from build123d import *

# Parameters (mm, degrees)
SKETCH1_R           = 2.66
BOSS_EXTRUDE1_DEPTH = 3
CUT_EXTRUDE1_DEPTH  = 2
SKETCH3_R           = 1.5
BOSS_EXTRUDE2_DEPTH = 10


with BuildPart() as part:
    # Sketch1 → Boss-Extrude1 (new body)
    with BuildSketch(Plane(origin=(0, 0, 0), x_dir=(1, 0, 0), z_dir=(0, 1, 0))):
        with Locations(Location((0, 0, 0), (0, 0, 270))):
            Circle(SKETCH1_R)
    extrude(amount=BOSS_EXTRUDE1_DEPTH)

    # Sketch2 → Cut-Extrude1 (cut)
    with BuildSketch(Plane(origin=(0, 3, 0), x_dir=(1, 0, 0), z_dir=(0, 1, 0))):
        Polygon((1.732050808, 0), (0.866025404, 1.5), (-0.866025404, 1.5), (-1.732050808, 0), (-0.866025404, -1.5), (0.866025404, -1.5), align=None)
    extrude(amount=-CUT_EXTRUDE1_DEPTH, mode=Mode.SUBTRACT)

    # Sketch3 → Boss-Extrude2 (add)
    with BuildSketch(Plane.XZ):
        with Locations(Location((0, 0, 0), (0, 0, 90))):
            Circle(SKETCH3_R)
    extrude(amount=BOSS_EXTRUDE2_DEPTH)


solid = part.part
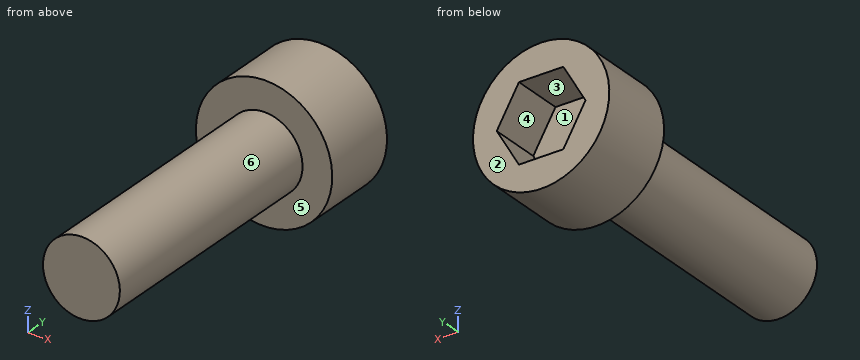
The listing builds one solid part. Answer for the finished solid, in the listing's coordinates (mm). Face numbers are marked on the shaded views. A direction names the side the tool comes from. Coordinates: 2 decimals unless noted, no trailing zeros. Loops run counter-clockwise (first coordinate to the right, second up) from the corner with the lowest first, then second, coordinate; pieces in that order, holes last.
1) Find section D-D on y = -5.5. Write down the section's boundary in (x, z).
2) Find section B-B on y = 1.75. Write down the section's boundary in (x, z).
3) Flat-ended cylindrical pins translate along their axes: pin 1 Ø0.9 at (x, z) = (0, -0.5) entering from +Y; pin 2 Ø1 at (y, z) = (-6.5, 1) entering from -X; pin 3 Ø1 at (x, z) = (-1, -1) entering from +Y; pin 4 Ø0.5 at (x, y) = (-0.5, 2) entering from +Z. Find the tip coordinate at first contact, or state that the pin passes through.
4) Find section A-A on x = 0. Write down the section's boundary in (y, z), then the cut area to 3 significant figures.
5) A tool of negligible diameter and unlimited length cuts with its end or side. For the marked faces 1 and 2, from which of +Z, -Z, +X, -X, +Y, -Y can it reach the whole face along a straight path? Write none if from no direction.
6) Find section C-C on z = 1.2. Write down the section's boundary in (x, y), then the cut area to 3 significant figures.
7) Determine the mould class of the marked faces 3, 4, 5 and 6 for opening direction X: pulls with the +X half, pulls with the -X half, needs draft (parallel to the pull), parting line crosses it, or undercut.
8) Find the intervals of material crossed by L1, parallel to Z at x = -0.3, y = 1.25; L2, parallel to Z at x = -0.1, y = -5.75; L3, parallel to Y at x = 1.25, z = -1, in increasing order.
Values:
1. outline: circle Ø3 at (0, 0)
2. outline: circle Ø5.32 at (0, 0); hole (-1.73, 0) - (-0.87, -1.5) - (0.87, -1.5) - (1.73, 0) - (0.87, 1.5) - (-0.87, 1.5) - close
3. pin 1: stops at y = 1
3. pin 2: stops at x = -1.41
3. pin 3: stops at y = 3
3. pin 4: stops at z = 2.65
4. outline: (-10, -1.5) - (0, -1.5) - (0, -2.66) - (3, -2.66) - (3, -1.5) - (1, -1.5) - (1, 1.5) - (3, 1.5) - (3, 2.66) - (0, 2.66) - (0, 1.5) - (-10, 1.5) - close
4. area: 40.0 mm2
5. face 1: +Y
5. face 2: +Z, -Z, +X, -X, +Y
6. outline: (-2.37, 0) - (-0.9, 0) - (-0.9, -10) - (0.9, -10) - (0.9, 0) - (2.37, 0) - (2.37, 3) - (1.04, 3) - (1.04, 1) - (-1.04, 1) - (-1.04, 3) - (-2.37, 3) - close
6. area: 28.1 mm2
7. face 3: undercut
7. face 4: undercut
7. face 5: needs draft
7. face 6: parting line crosses it
8. L1: z = -2.64 to -1.5, 1.5 to 2.64
8. L2: z = -1.5 to 1.5
8. L3: y = 0 to 3
